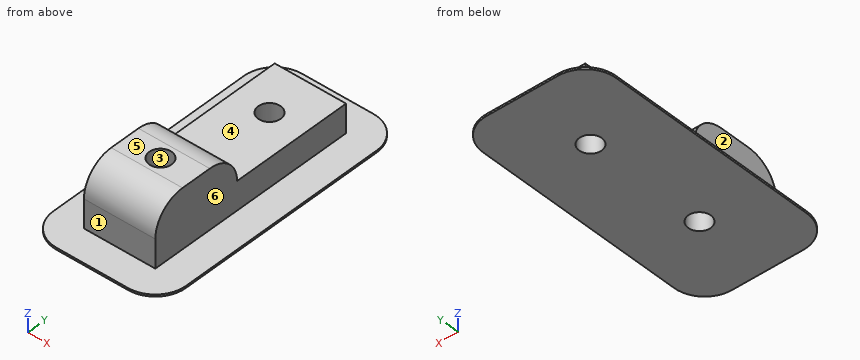
```python
from build123d import *

# Parameters (mm, degrees)
F1_DEPTH = 7
F2_R     = 2.99999
F3_R     = 1.1
F4_DEPTH = 6.001
F5_W     = 7
F5_H     = 21
F6_DEPTH = 0.2


# Not quite as in the source:
# - a fillet or chamfer is up to 0.001 mm smaller than in the source, because OpenCascade refuses the exact size


with BuildPart() as f1:
    # F0 (on Right) → F1 (new body)
    with BuildSketch(Plane.YZ):
        Polygon((-21, 0), (0, 0), (0, 3), (-12, 3), (-12, 6), (-21, 6), align=None)
    extrude(amount=F1_DEPTH)

    # F2 (radius 3 in the source; OpenCascade refuses exactly that, so slightly less here)
    f2_edges = [f1.edges().sort_by_distance(p)[0] for p in [
        (3.5, -12, 6),
        (3.5, -21, 6),
    ]]
    fillet(f2_edges, radius=F2_R)

    # F3 (on face) → F4 (cut, through all)
    with BuildSketch(Plane(origin=(0, 0, 0), x_dir=(1, 0, 0), z_dir=(0, 0, -1))):
        with Locations((3.5, 16.5)):
            Circle(F3_R)
        with Locations((3.5, 4.5)):
            Circle(F3_R)
    extrude(amount=-F4_DEPTH, mode=Mode.SUBTRACT)

    # F5 (on face) → F6 (join)
    with BuildSketch(Plane(origin=(0, 0, 0), x_dir=(1, 0, 0), z_dir=(0, 0, -1))):
        with BuildLine():
            ThreePointArc((0, 24), (-2.1213203436, 23.1213203436), (-3, 21))
            Line((-3, 21), (-3, 0))
            ThreePointArc((-3, 0), (-2.1213203436, -2.1213203436), (0, -3))
            Line((0, -3), (7, -3))
            ThreePointArc((7, -3), (9.1213203436, -2.1213203436), (10, 0))
            Line((10, 0), (10, 21))
            ThreePointArc((10, 21), (9.1213203436, 23.1213203436), (7, 24))
            Line((7, 24), (0, 24))
        make_face()
        with Locations((3.5, 10.5)):
            Rectangle(F5_W, F5_H, mode=Mode.SUBTRACT)
    extrude(amount=-F6_DEPTH)


solid = f1.part
```
For this review, take the finished solid that the model builds, in its own axes (mm). Face numbers are marked on the shaded views. A direction names the side the tool comes from. Round coordinates to 2 decimals unless told otherwise and drop trailing zeros. Write each loop counter-clockwise with the first axis right and the second up, starting at its lowest first coordinate (ties: lowest second). Pieces come first, ordered by that corner, then holes. Notation, with made-up numbers: (8, 29) - (20, 29) arc R31 ccw to (20, 54) - close; hole circle Ø4 at (62.25, 35). An arc over 180 degrees is marked (long way). Write each question's results on one line, items separated by ' | '.
Item 1: Take a section at B-B on y = -4.5. State the section outline as (x, z) points.
Calculated:
outline: (-3, 0) - (2.4, 0) - (2.4, 3) - (0, 3) - (0, 0.2) - (-3, 0.2) - close; (4.6, 0) - (10, 0) - (10, 0.2) - (7, 0.2) - (7, 3) - (4.6, 3) - close
Item 2: Take a section at A-A on x = 3.5. Count the separate pieces of the cut face and the enclosed holes in it, then the cut area to 3 significant figures.
Calculated:
separate pieces: 3 | enclosed holes: 0 | area: 67.5 mm^2
Item 3: Take a section at D-D on z = 1.3. State the section outline as (x, y) points, then the cut area to 3 significant figures.
Calculated:
outline: (0, -21) - (7, -21) - (7, 0) - (0, 0) - close; hole circle Ø2.2 at (3.5, -16.5); hole circle Ø2.2 at (3.5, -4.5) | area: 139 mm^2
Item 4: For pin 1 (4 mm diameter, centred on x = 5, y = -7.5, fed in from +Z); pin 2 (1.7 mm diameter, centred on y = -9.5, z = 3.5, fed in from -X); pin 3 (0.8 mm diameter, centred on x = 4, z = 1.5, fed in from -Y); pin 4 (3 mm diameter, centred on x = 3.5, y = -16.5, fed in from -Z), all flat-tipped, find the tip position at first contact; note any pin that passes through.
Calculated:
pin 1: stops at z = 3 | pin 2: stops at x = 0 | pin 3: stops at y = -21 | pin 4: stops at z = 0
Item 5: To check wall thickness, follow line 1 along Y through (x, z) = (3.5, 0.75); line 2 along X through (y, z) = (-4.5, 1.8); line 3 along Y through (x, z) = (3.5, 3.1). State the ranges of each line that lie inside material, in increasing order. Write a range as from..to.
Calculated:
line 1: y = -21..-17.6, -15.4..-5.6, -3.4..0 | line 2: x = 0..2.4, 4.6..7 | line 3: y = -21..-17.6, -15.4..-12
Item 6: For the marked faces 4, 5 and 6, list the 3-axis set-ups (+Z, -Z, +X, -X, +Y, -Y) from which the entire face can be reached by the end or side of a thin tool; tool diameter is ignored.
Calculated:
face 4: +Z, +X, -X, +Y | face 5: +Z, +X, -X, +Y, -Y | face 6: +Z, +X, +Y, -Y
Item 7: Draft analysis for pull direction Y (two halves, no side actions). For the marked faces 1, 2 and 3, state which applies: pulls with the +Y half, pulls with the -Y half, needs draft (parallel to the pull), parting line crosses it, or undercut.
Calculated:
face 1: pulls with the -Y half | face 2: needs draft | face 3: undercut
